Read the model definition and answer for the solid it produces. Units are mm, in the model's axes. A direction names the side the tool comes from. Give positions to 0.01 mm unless a question says otherwise; leave off trailing zeros. Write item = value, one per line.
from build123d import *

# Parameters (mm, degrees)
SKETCH1_R                 = 6.35
SKETCH1_R_2               = 5.2832
PIPE_0_5_SCH_40_1_DEPTH   = 175.328598267
SKETCH1_ON_SEGMENT_2_R    = 6.35
SKETCH1_ON_SEGMENT_2_R_2  = 5.2832
PIPE_0_5_SCH_40_1_2_ANGLE = 90
SKETCH1_ON_SEGMENT_3_R    = 6.35
SKETCH1_ON_SEGMENT_3_R_2  = 5.2832
PIPE_0_5_SCH_40_1_3_DEPTH = 116.982148253
SKETCH1_ON_SEGMENT_4_R    = 6.35
SKETCH1_ON_SEGMENT_4_R_2  = 5.2832
PIPE_0_5_SCH_40_1_4_ANGLE = 90
SKETCH1_ON_SEGMENT_5_R    = 6.35
SKETCH1_ON_SEGMENT_5_R_2  = 5.2832
PIPE_0_5_SCH_40_1_5_DEPTH = 50.697047229


with BuildPart() as part:
    # Sketch1 → Pipe 0.5 SCH 40(1) (new body)
    with BuildSketch(Plane(origin=(-440.41650414, 719.319181201, 431.8), x_dir=(1, 0, 0), z_dir=(0, -1, 0))):
        Circle(SKETCH1_R)
        Circle(SKETCH1_R_2, mode=Mode.SUBTRACT)
    extrude(amount=PIPE_0_5_SCH_40_1_DEPTH)


with BuildPart() as body_2:
    # Sketch1 on segment 2 (carried to the start of arc 2) → Pipe 0.5 SCH 40_1 2 (revolve)
    with BuildSketch(Plane(origin=(-440.41650414, 543.990582935, 431.8), x_dir=(1, 0, 0), z_dir=(0, -1, 0))):
        Circle(SKETCH1_ON_SEGMENT_2_R)
        Circle(SKETCH1_ON_SEGMENT_2_R_2, mode=Mode.SUBTRACT)
    revolve(axis=Axis((-390.908254533, 543.990582935, 443.183023362), (-0.224075263, 0, 0.974571843)), revolution_arc=PIPE_0_5_SCH_40_1_2_ANGLE)


with BuildPart() as body_3:
    # Sketch1 on segment 3 (carried to segment 3) → Pipe 0.5 SCH 40_1 3 (new body)
    with BuildSketch(Plane(origin=(-390.908254533, 493.190582935, 443.183023362), x_dir=(0.050209724, 0.974571843, -0.218377442), z_dir=(0.974571843, 0, 0.224075263))):
        Circle(SKETCH1_ON_SEGMENT_3_R)
        Circle(SKETCH1_ON_SEGMENT_3_R_2, mode=Mode.SUBTRACT)
    extrude(amount=PIPE_0_5_SCH_40_1_3_DEPTH)


with BuildPart() as body_4:
    # Sketch1 on segment 4 (carried to the start of arc 4) → Pipe 0.5 SCH 40_1 4 (revolve)
    with BuildSketch(Plane(origin=(-276.900746752, 493.190582935, 469.395829002), x_dir=(0.050209724, 0.974571843, -0.218377442), z_dir=(0.974571843, 0, 0.224075263))):
        Circle(SKETCH1_ON_SEGMENT_4_R)
        Circle(SKETCH1_ON_SEGMENT_4_R_2, mode=Mode.SUBTRACT)
    revolve(axis=Axis((-276.882509946, 442.39064813, 469.316511553), (0.224074975, 0.001602106, -0.974570592)), revolution_arc=PIPE_0_5_SCH_40_1_4_ANGLE)


with BuildPart() as body_5:
    # Sketch1 on segment 5 (carried to segment 5) → Pipe 0.5 SCH 40_1 5 (new body)
    with BuildSketch(Plane(origin=(-227.374260339, 442.39064813, 480.699534915), x_dir=(0.999999936, 0.000358992, 2.8e-07), z_dir=(0.000358992, -0.999998717, -0.001561367))):
        Circle(SKETCH1_ON_SEGMENT_5_R)
        Circle(SKETCH1_ON_SEGMENT_5_R_2, mode=Mode.SUBTRACT)
    extrude(amount=PIPE_0_5_SCH_40_1_5_DEPTH)


with BuildPart() as part_1:
    add(part.part)

    # Pipe 0.5 SCH 40(1) as one body: union body 2, body 3, body 4, body 5
    add(body_2.part)
    add(body_3.part)
    add(body_4.part)
    add(body_5.part)


solid = part_1.part
(1) A tool of negligible diameter and unlimited length cuts with its end or side. For faces 4 (the cylindrical face through (-334.796, 498.457, 456.513)), 5 (the cylindrical face through (-441.79, 632.88, 425.6)), from which of +Z, -Z, +X, -X, +Y, -Y can it reach the whole face along a straight path? Write none if from no direction.
Checks:
face_4 = none
face_5 = +Y
(2) Consider L1, parallel to Y at x = -359, z = 450.5. Determine where the line is inside the solid, lowest interval first.
Checks:
L1 = 486.84 to 487.91, 498.47 to 499.54
(3) For a pull along X with two mould halves and no side action, classify faces 1 (the cylindrical face through (-221.5, 417.4, 478.23)), 2 (the flat face through (-443, 719.319, 437)), 3 (the cylindrical face through (-435.536, 632.882, 429.777)) as released by +X, released by -X, zero draft, split by the parting line, or undercut.
Checks:
face_1 = split by the parting line
face_2 = zero draft
face_3 = undercut
